Read the model definition and answer for the solid it produces. Units are mm, in the model's axes. Face numbers are marked on the shaded views. A direction names the side the tool comes from. Give positions to 0.01 mm unless a question says otherwise; leave off trailing zeros. Write each loop counter-clockwise with the first axis right and the second up, starting at its lowest first coordinate (ties: lowest second). Pieces come first, ordered by that corner, then holes. Notation, with made-up numbers: M -14,21.25 L 8,21.25 A32 ccw 8,57.25 Z; hole C 55.5,27 d4. An arc over 180 degrees is marked long. Answer as CSV lines item,"result". Start each with the question number.
```python
from build123d import *

# Parameters (mm, degrees)
F0_W     = 88.9
F0_H     = 152.4
F1_DEPTH = 50.8
F2_W     = 82.55
F2_H     = 28.864218
F2_H_2   = 32.227332
F2_H_3   = 33.203915
F2_H_4   = 34.661213
F3_DEPTH = 88.9
F4_R     = 5.08


with BuildPart() as f1:
    # F0 (on Front) → F1 (new body, symmetric)
    with BuildSketch(Plane.XZ):
        Rectangle(F0_W, F0_H)
    extrude(amount=F1_DEPTH, both=True)

    # F2 (on face) → F3 (cut)
    with BuildSketch(Plane.XZ.offset(50.8)):
        with Locations((0, 55.417891)):
            Rectangle(F2_W, F2_H)
        with Locations((0, 22.332116)):
            Rectangle(F2_W, F2_H_2)
        with Locations((0, -14.485167)):
            Rectangle(F2_W, F2_H_3)
        with Locations((0, -52.519393)):
            Rectangle(F2_W, F2_H_4)
    extrude(amount=-F3_DEPTH, mode=Mode.SUBTRACT)

    # F4
    f4_edges = [f1.edges().sort_by_distance(p)[0] for p in [
        (-44.45, 0, 76.2),
        (44.45, 0, 76.2),
        (0, 50.8, 76.2),
        (0, -50.8, 76.2),
        (-41.275, -6.35, 38.445782),
        (41.275, -6.35, 38.445782),
        (41.275, -6.35, 69.85),
        (-41.275, -6.35, 69.85),
    ]]
    fillet(f4_edges, radius=F4_R)


solid = f1.part
```
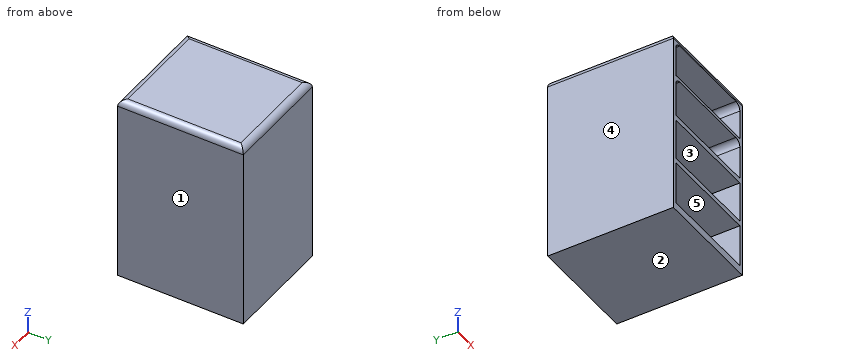
1. Find section C-C on x = 18. Determine the outline of the cut face in (y, z).
2. Find section A-A on y = -2. Determine the outline of the cut face in (x, z) (3 decimals), then the cut area to 3 significant figures.
3. Given pin 1 (14.5 mm diameter, centred on x = 10.5, z = 55, fed in from -Y), flat-ended and moving along its own axis, determine where the tip first touches the part or whether it passes through.
4. Find section B-B on z = 21.5. Determine the outline of the cut face in (x, y) (3 decimals), then the cut area to 3 significant figures.
5. For the marked faces 4 and 5, determine the directions among +Z, -Z, +X, -X, +Y, -Y from which every point of the face is accessible in a straight line to the end or side of a thin tool.
6. Find the intervals of material crossed by line 1 (Z direction, x = -28, y = -28); line 2 (X direction, y = 31.5, z = -1.5) (3 decimals); line 3 (Y direction, x = -23, z = 62), in increasing order. Write a range as [from, to].
7. Determine the mould class of the marked faces 1, 2 and 3 for opening direction X: +X half, -X half, draft (parallel to the pull), parting line (faces both ways), or undercut.
Computed:
1,outline,"M -50.8,-76.2 L 50.8,-76.2 L 50.8,71.12 A5.08 ccw 45.72,76.2 L -45.72,76.2 A5.08 ccw -50.8,71.12 L -50.8,69.85 L 38.1,69.85 L 38.1,40.99 L -50.8,40.99 L -50.8,38.45 L 38.1,38.45 L 38.1,6.22 L -50.8,6.22 L -50.8,2.12 L 38.1,2.12 L 38.1,-31.09 L -50.8,-31.09 L -50.8,-35.19 L 38.1,-35.19 L 38.1,-69.85 L -50.8,-69.85 Z"
2,outline,"M -44.45,-76.2 L 44.45,-76.2 L 44.45,71.12 A5.08 ccw 39.37,76.2 L -39.37,76.2 A5.08 ccw -44.45,71.12 Z; hole M -41.275,-69.85 L 41.275,-69.85 L 41.275,-35.189 L -41.275,-35.189 Z; hole M -41.275,-31.087 L 41.275,-31.087 L 41.275,2.117 L -41.275,2.117 Z; hole M -41.275,6.218 L 41.275,6.218 L 41.275,33.366 A5.08 ccw 36.195,38.446 L -36.195,38.446 A5.08 ccw -41.275,33.366 Z; hole M -41.275,40.986 L 41.275,40.986 L 41.275,64.77 A5.08 ccw 36.195,69.85 L -36.195,69.85 A5.08 ccw -41.275,64.77 Z"
2,area,"2,910 mm^2"
3,pin 1,"stops at y = 38.1"
4,outline,"M -44.45,-50.8 L -41.275,-50.8 L -41.275,38.1 L 41.275,38.1 L 41.275,-50.8 L 44.45,-50.8 L 44.45,50.8 L -44.45,50.8 Z"
4,area,"1,690 mm^2"
5,face 4,"+Z, -Z, -X, +Y, -Y"
5,face 5,"-Y"
6,line 1,"z = [-76.2, -69.85], [-35.19, -31.09], [2.12, 6.22], [38.45, 40.99], [69.85, 76.2]"
6,line 2,"x = [-44.45, -41.275], [41.275, 44.45]"
6,line 3,"y = [38.1, 50.8]"
7,face 1,"+X half"
7,face 2,"draft"
7,face 3,"undercut"
